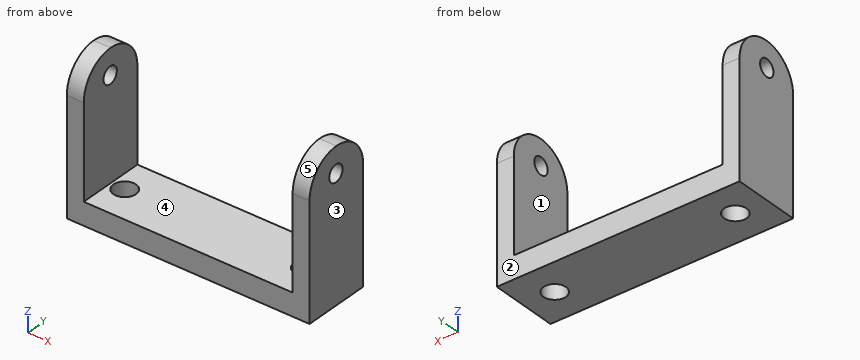
Autodesk Inventor part; units mm, degrees
ref_plane "YZ Plane" through (0, 0, 0) normal (1, 0, 0) x (0, 1, 0)
ref_plane "XZ Plane" through (0, 0, 0) normal (0, 1, 0) x (-1, 0, 0)
ref_plane "XY Plane" through (0, 0, 0) normal (0, 0, 1) x (1, 0, 0)
sketch "Szkic1" plane through (0, 0, 0) normal (0, 0, 1) x (1, 0, 0)
  line L0 (0, 0) -> (-32, 0)
  circle A0 centre (-32, 0) radius 2
  circle A1 centre (0, 0) radius 2
  line L1 (-37.5, -6) -> (5.5, -6)
  line L2 (5.5, -6) -> (5.5, 6)
  line L3 (5.5, 6) -> (-37.5, 6)
  line L4 (-37.5, 6) -> (-37.5, -6)
  line L5 (-37.5, -6) -> (5.5, 6) construction
  line L6 (5.5, -6) -> (-37.5, 6) construction
  point P0 (-16, 0)
  dimension "d2" = 32
  dimension "d3" = 4
  dimension "d4" = 4
  dimension "d5" = 43
  dimension "d6" = 12
extrude "Wyciągnięcie proste1" add sketch "Szkic1" along normal blind 4
sketch "Szkic2" plane through (0, 0, 4) normal (0, 0, 1) x (1, 0, 0)
  line L0 (5.5, -6) -> (5.5, 6)
  line L1 (-37.5, -6) -> (5.5, -6)
  line L2 (5.5, 6) -> (2.5, 6)
  line L3 (2.5, 6) -> (2.5, -6)
  line L4 (2.5, -6) -> (5.5, -6)
  line L5 (5.5, -6) -> (5.5, 6)
  line L6 (-37.5, 6) -> (-34.5, 6)
  line L7 (-34.5, 6) -> (-34.5, -6)
  line L8 (-34.5, -6) -> (-37.5, -6)
  line L9 (-37.5, -6) -> (-37.5, 6)
  dimension "d12" = 3
  dimension "d13" = 3
extrude "Wyciągnięcie proste2" add sketch "Szkic2" along normal blind 22.5
fillet "Zaokrąglenie1" radius 6 4 edges at (-36, 6, 26.5) (-36, -6, 26.5) (4, 6, 26.5) (4, -6, 26.5)
sketch "Szkic3" plane through (-34.5, -6, 4) normal (1, 0, 0) x (0, 0, -1)
  line L0 (0, 5.9057) -> (-18, 5.9057)
  circle A0 centre (-18, 5.9057) radius 1.5
  point P0 (4, 6)
  dimension "d15" = 18
  dimension "d21" = 3
extrude "Wyciągnięcie proste3" cut sketch "Szkic3" along normal mid plane 100
properties part number "Zebatka holderv2"
Geometry check sheet. Reference: the model listing, model coordinates, mm. Face numbers are marked on the shaded views. A direction names the side the tool comes from. Coordinates: 2 decimals unless noted, no trailing zeros. Order: outer loops, then holes, each group sorted by start corner. A loop starts at its lowest first (then second) coordinate and runs counter-clockwise, first axis right, second up.
Q1. Thickness scan on probe 1 along X at (y, z) = (5.5, 11.25); probe 2 along Z at (x, y) = (-7, 4); probe 3 along X at (y, z) = (0.25, 1.5). Record the ranges inside material, lowest first.
Reply:
probe 1: x = -37.5 to -34.5, 2.5 to 5.5
probe 2: z = 0 to 4
probe 3: x = -37.5 to -33.98, -30.02 to -1.98, 1.98 to 5.5
Q2. Sectioned sample at B-B on z = 22. Record the cut outline in (x, y), and give its area (3 significant figures).
Reply:
outline: (-37.5, -5.81) - (-34.5, -5.81) - (-34.5, -1.59) - (-37.5, -1.59) - close; (-37.5, 1.41) - (-34.5, 1.41) - (-34.5, 5.81) - (-37.5, 5.81) - close; (2.5, -5.81) - (5.5, -5.81) - (5.5, -1.59) - (2.5, -1.59) - close; (2.5, 1.41) - (5.5, 1.41) - (5.5, 5.81) - (2.5, 5.81) - close
area: 51.7 mm2
Q3. Depth check by flat-ended pin: pin 1 Ø3 at (x, z) = (0, 8) entering from -Y; pin 2 Ø6 at (x, y) = (-26.5, 1) entering from +Z. Enter the tip coordinate at first touch or a pass-through.
Reply:
pin 1: passes through
pin 2: stops at z = 4
Q4. Sectioned sample at D-D on y = -1. Record the cut outline in (x, z).
Reply:
outline: (-37.5, 0) - (-33.73, 0) - (-33.73, 4) - (-34.5, 4) - (-34.5, 20.8) - (-37.5, 20.8) - close; (-37.5, 23.2) - (-34.5, 23.2) - (-34.5, 26.42) - (-37.5, 26.42) - close; (-30.27, 0) - (-1.73, 0) - (-1.73, 4) - (-30.27, 4) - close; (1.73, 0) - (5.5, 0) - (5.5, 20.8) - (2.5, 20.8) - (2.5, 4) - (1.73, 4) - close; (2.5, 23.2) - (5.5, 23.2) - (5.5, 26.42) - (2.5, 26.42) - close
Q5. Draft check along X on the marked faces 3, 4 and 5. Enter one of: released by +X, released by -X, zero draft, split by the parting line, or undercut.
Reply:
face 3: released by +X
face 4: undercut
face 5: zero draft
Q6. Sectioned sample at A-A on x = -32. Record the cut outline in (y, z).
Reply:
outline: (-6, 0) - (-2, 0) - (-2, 4) - (-6, 4) - close; (2, 0) - (6, 0) - (6, 4) - (2, 4) - close
Q7. Tool access check on the marked faces 1 and 2. Record the directions out of +Z, -Z, +X, -X, +Y, -Y that give a thin tool (end or side, any length) a straight path to the whole face; none if there is none.
Reply:
face 1: +Z, +Y, -Y
face 2: +Z, -Z, +X, -X, +Y
Q8. Sectioned sample at C-C on z = 18.75. Record the cut outline in (x, y).
Reply:
outline: (-37.5, -6) - (-34.5, -6) - (-34.5, 6) - (-37.5, 6) - close; (2.5, -6) - (5.5, -6) - (5.5, 6) - (2.5, 6) - close
